Can you work these out from the drawing? Everything is in mm from the part's minimum corner. Give positions to 0.01 mm unless a question says otherwise; leave off trailing zeros. Order: outer loops, then holes, each group sorted by start corner. A loop starts at its lowest first (then second) coordinate and runs counter-clockwise, first axis right, second up. Notation, with made-up numbers: (19.25, 1.25) - (62.25, 1.25) arc R5 ccw to (62.25, 10.25) - close; hole circle Ø1 at (67.5, 29.5). An arc over 180 degrees is marked (long way). Answer as a JSON object with one key per item and string values.
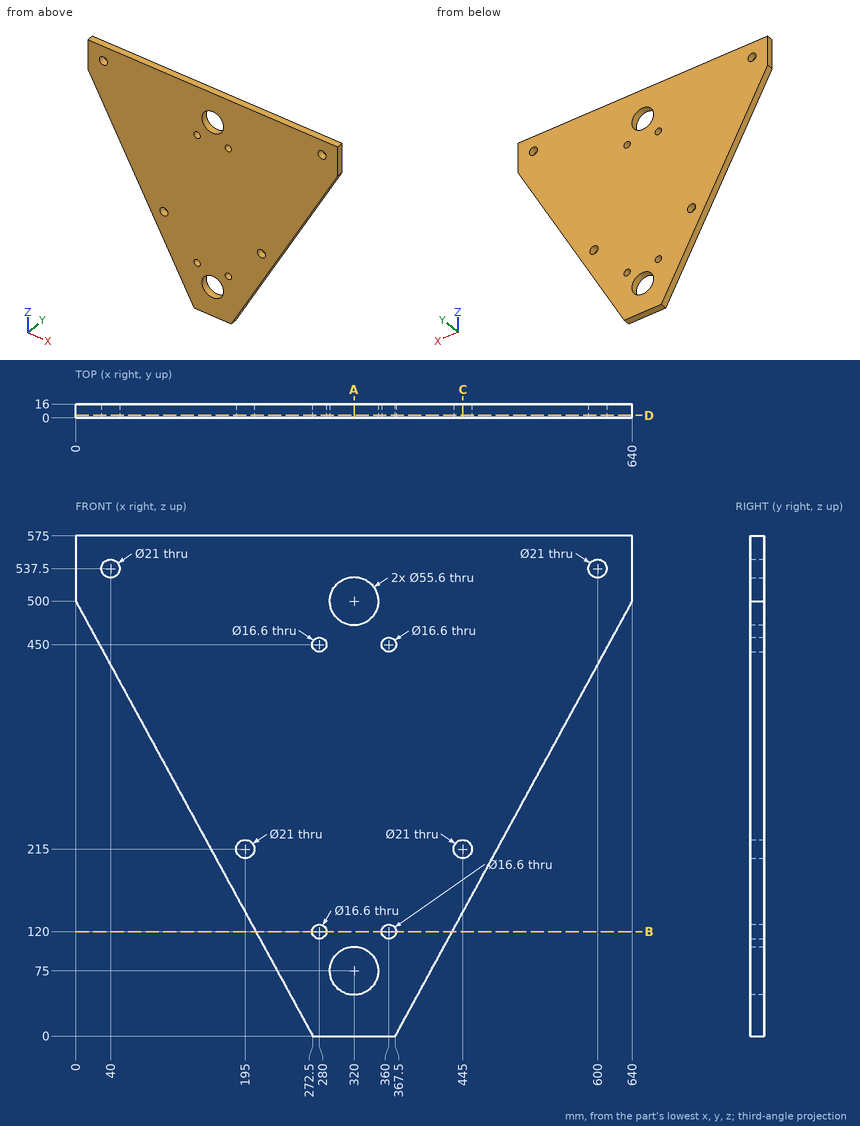
Q1. If we section it at D-D, the plane y = 3: Count the separate pieces of the cut face and the enclosed holes in it, then the cut area to 3 significant figures.
Recorded:
{"separate pieces": "1", "enclosed holes": "10", "area": "225,000 mm^2"}
Q2. If we section it at C-C, the plane x = 445: Please give me the cut outline in (y, z), then the cut area to 3 significant figures.
Recorded:
{"outline": "(0, 142.2) - (16, 142.2) - (16, 204.5) - (0, 204.5) - close; (0, 225.5) - (16, 225.5) - (16, 575) - (0, 575) - close", "area": "6,590 mm^2"}
Q3. If we section it at A-A, the plane x = 320: Please give me the cut outline in (y, z), then the cut area to 3 significant figures.
Recorded:
{"outline": "(0, 0) - (16, 0) - (16, 47.2) - (0, 47.2) - close; (0, 102.8) - (16, 102.8) - (16, 472.2) - (0, 472.2) - close; (0, 527.8) - (16, 527.8) - (16, 575) - (0, 575) - close", "area": "7,420 mm^2"}
Q4. I'm going to push flat-ended pins straight in: pin 1 Ø19 at (x, z) = (280, 450) entering from -Y; pin 2 Ø3 at (y, z) = (11.5, 297) entering from +X; pin 3 Ø2 at (y, z) = (9.5, 269) entering from +X; pin 4 Ø5 at (y, z) = (9, 426.5) entering from -X (3 decimals). Where does each tip first touch, or does it pass through?
Recorded:
{"pin 1": "stops at y = 0", "pin 2": "stops at x = 530.18", "pin 3": "stops at x = 514.65", "pin 4": "stops at x = 38.695"}
Q5. I need wall thicknesses on L1, parallel to X at y = 12.5, z = 537.5; L2, parallel to X at y = 2.25, z = 221 (3 decimals); L3, parallel to Z at x = 602.5, y = 9.5. Which ranges of each line are inside material? Lowest first, please.
Recorded:
{"L1": "x = 0 to 29.5, 50.5 to 589.5, 610.5 to 640", "L2": "x = 152.055 to 186.383, 203.617 to 436.383, 453.617 to 487.945", "L3": "z = 431.19 to 527.3, 547.7 to 575"}
Q6. If we section it at B-B, the plane z = 120: Please give me the cut outline in (x, y).
Recorded:
{"outline": "(207.1, 0) - (271.7, 0) - (271.7, 16) - (207.1, 16) - close; (288.3, 0) - (351.7, 0) - (351.7, 16) - (288.3, 16) - close; (368.3, 0) - (432.9, 0) - (432.9, 16) - (368.3, 16) - close"}
